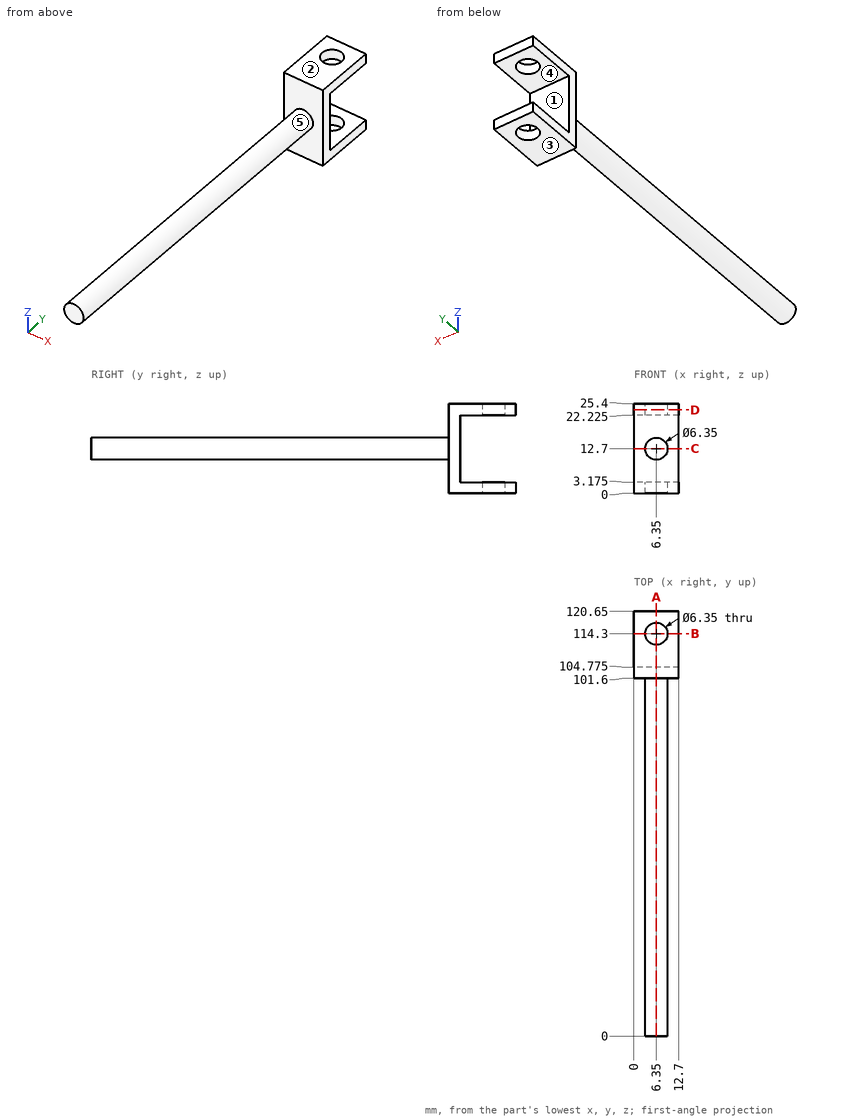
Verification items for this drawing (mm, ordinates from the low corner). A direction names the side the tool comes from. Give positions to 0.01 mm unless a question says otherwise; leave off trailing zeros. Loops run counter-clockwise (first coordinate to the right, second up) from the corner with the lowest first, then second, coordinate; pieces in that order, holes last. Notation, with made-up numbers: M 12,61 L 50,61 A22 ccw 50,81 Z; hole C 38,53 d3. An arc over 180 degrees is marked long. Answer as a JSON object with one key per item and string values. Group by question number.
Item 1: Sectioned sample at D-D on z = 23.75. Record the boundary of the cut face in (x, y) (3 decimals).
Item 2: Sectioned sample at B-B on y = 114.3. Record the boundary of the cut face in (x, z) (3 decimals), plus the area to 3 significant figures.
Item 3: Mould release check, pull along Z, two halves, no side actions. Record for the marked faces 1, 2 and 3: pulls with the +Z half, pulls with the -Z half, needs draft (parallel to the pull), parting line crosses it, or undercut.
Item 4: Sectioned sample at A-A on x = 6.35. Record the boundary of the cut face in (y, z) (3 decimals), plus the area to 3 significant figures.
Item 5: Gauge pin test, flat ends, axial feed: pin 1 (6 mm diameter, centred on x = 5, z = 22.5, fed in from -Y); pin 2 (4 mm diameter, centred on x = 6.35, y = 114.3, fed in from +Z); pin 3 (1 mm diameter, centred on x = 7, z = 6.5, fed in from +Y) (3 decimals); pin 4 (1 mm diameter, centred on y = 91, z = 9.5, fed in from -X). Record the tip position at first contact, or that the pin passes through.
Item 6: Sectioned sample at C-C on z = 12.7. Record the boundary of the cut face in (x, y) (3 decimals), plus the area to 3 significant figures.
Item 7: Access from +Z, -Z, +X, -X, +Y, -Y to the whole of each face (thin tool, end or side, straight path). Record for the marked faces 4 and 5.
Item 8: Material ranges on L1, parallel to Y at x = 6.35, z = 24.3 (3 decimals); L2, parallel to Y at x = 10.5, z = 19 (3 decimals); L3, parallel to Y at x = 9.75, z = 23.25, recorded low to high.
Findings below:
{
 "1": {"outline": "M 0,101.6 L 12.7,101.6 L 12.7,120.65 L 0,120.65 Z; hole C 6.35,114.3 d6.35"},
 "2": {"outline": "M 0,0 L 3.175,0 L 3.175,3.175 L 0,3.175 Z; M 0,22.225 L 3.175,22.225 L 3.175,25.4 L 0,25.4 Z; M 9.525,0 L 12.7,0 L 12.7,3.175 L 9.525,3.175 Z; M 9.525,22.225 L 12.7,22.225 L 12.7,25.4 L 9.525,25.4 Z", "area": "40.3 mm2"},
 "3": {"face 1": "undercut", "face 2": "pulls with the +Z half", "face 3": "pulls with the -Z half"},
 "4": {"outline": "M 0,9.525 L 101.6,9.525 L 101.6,0 L 111.125,0 L 111.125,3.175 L 104.775,3.175 L 104.775,22.225 L 111.125,22.225 L 111.125,25.4 L 101.6,25.4 L 101.6,15.875 L 0,15.875 Z; M 117.475,0 L 120.65,0 L 120.65,3.175 L 117.475,3.175 Z; M 117.475,22.225 L 120.65,22.225 L 120.65,25.4 L 117.475,25.4 Z", "area": "786 mm2"},
 "5": {"pin 1": "y = 101.6", "pin 2": "through", "pin 3": "y = 104.775", "pin 4": "x = 4.68"},
 "6": {"outline": "M 0,101.6 L 3.175,101.6 L 3.175,0 L 9.525,0 L 9.525,101.6 L 12.7,101.6 L 12.7,104.775 L 0,104.775 Z", "area": "685 mm2"},
 "7": {"face 4": "+X, -X, +Y", "face 5": "-Y"},
 "8": {"L1": "101.6 to 111.125, 117.475 to 120.65", "L2": "101.6 to 104.775", "L3": "101.6 to 120.65"}
}
